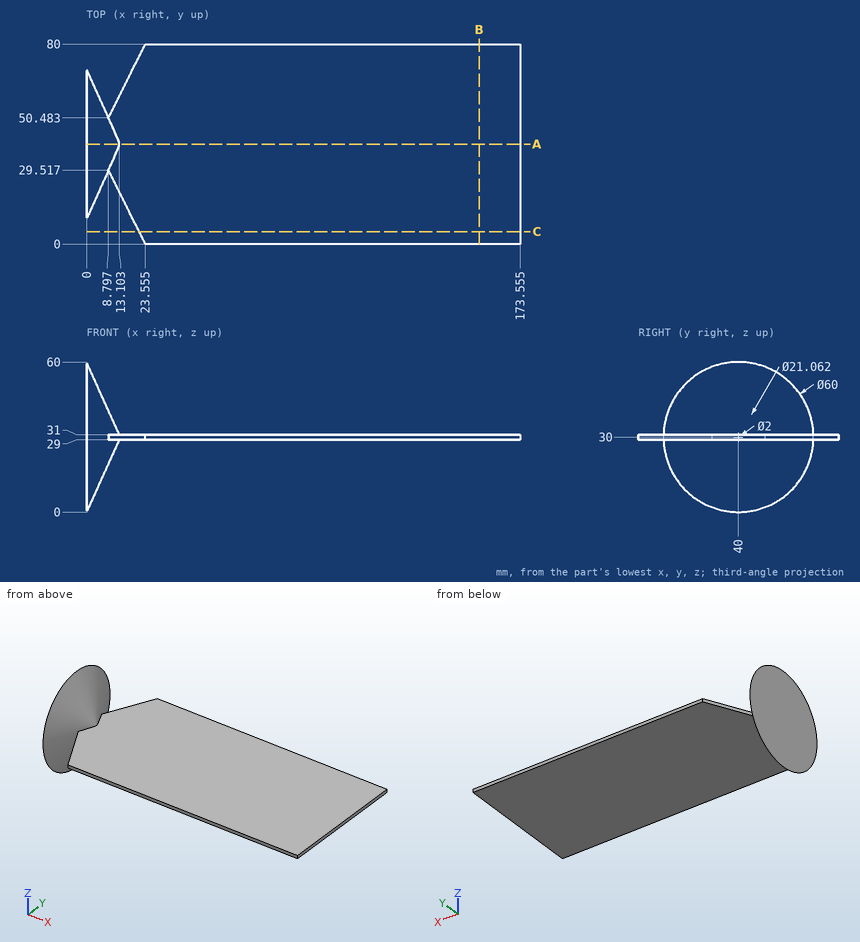
Study the drawing (mm; zero at the part's minimum x, y, z) and answer. Round coordinates to 2 decimals unless told otherwise and drop trailing zeros. Write each loop counter-clockwise with the first axis right and the second up, starting at its lowest first coordinate (ties: lowest second). Pieces come first, ordered by that corner, then holes. Notation, with made-up numbers: (48, 43.5) - (92, 43.5) arc R11 cw to (92, 48.5) - close; hole circle Ø4 at (-6, 57.25). An arc over 180 degrees is marked (long way). Use a Markdown table: item, result. Add a question column.
1. Flat-ended cylindrical pins translate along their axes: P1, Ø2, axis at y = 53.5, z = 11.5, coming from the +X side; P2, Ø1, axis at x = 105.5, y = 59, coming from the -Z side; P3, Ø5, axis at x = 74, y = 55.5, coming from the +Z side. Find the tip coordinate at first contact, or state that the pin passes through.
2. The part is cut by section A-A (y = 40). Write down the section's boundary in (x, z) (1 decimal).
3. The part is cut by section B-B (x = 157). Write down the section's boundary in (y, z), and give its area (3 significant figures).
4. The part is cut by section C-C (y = 5). Write down the section's boundary in (x, z) (1 decimal), and give its area (3 significant figures).
5. Consider line 1 (Z direction, x = 35, y = 30.5); line 2 (X direction, y = 41.5, z = 8.5); line 3 (X direction, y = 15.5, z = 17). Determine where each line is inside the solid, lowest interval first.
Reported:
| question | item | result |
|---|---|---|
| 1 | P1 | x = 3.66 |
| 1 | P2 | z = 29 |
| 1 | P3 | z = 31 |
| 2 | outline | (0, 0) - (13.1, 29) - (173.6, 29) - (173.6, 31) - (13.1, 31) - (0, 60) - close |
| 3 | outline | (0, 29) - (80, 29) - (80, 31) - (0, 31) - close |
| 3 | area | 160 mm^2 |
| 4 | outline | (21.1, 29) - (173.6, 29) - (173.6, 31) - (21.1, 31) - close |
| 4 | area | 305 mm^2 |
| 5 | line 1 | 29 to 31 |
| 5 | line 2 | 0 to 3.82 |
| 5 | line 3 | 0 to 1.02 |
